CAD build for the part. Positions are in the model's coordinates, mm. Face numbers are marked on the shaded views. Give positions to 0.01 mm unless a question says otherwise; leave off trailing zeros. Loops run counter-clockwise (first coordinate to the right, second up) from the corner with the lowest first, then second, coordinate; pieces in that order, holes last. Notation, with made-up numbers: M 8.5,34 L 46.5,34 A20 ccw 46.5,40 Z; hole C 38,8 d3. An arc over 180 degrees is marked long. Answer as CSV lines item,"result".
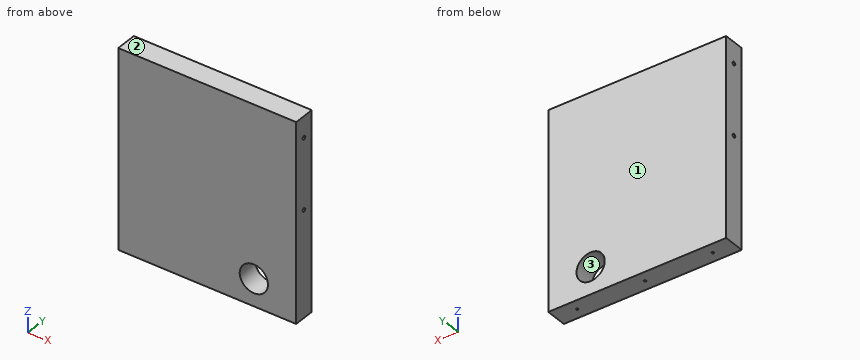
```python
from build123d import *

# Parameters (mm, degrees)
SKETCH1_W                  = 160.02
SKETCH1_H                  = 19.05
BOSS_EXTRUDE1_DEPTH        = 177.8
HOLE1_D                    = 1.98374
HOLE1_DEPTH                = 31.75
HOLE1_CSINK_D              = 10.16
HOLE1_CSINK_ANGLE          = 82
HOLE1_TIP                  = 0.595975622
HOLE3_D                    = 3.175
HOLE3_DEPTH                = 31.75
HOLE3_CSINK_D              = 10.16
HOLE3_CSINK_ANGLE          = 82
HOLE3_TIP                  = 0.953866233
HOLE4_D                    = 3.175
HOLE4_DEPTH                = 31.75
HOLE4_CSINK_D              = 10.16
HOLE4_CSINK_ANGLE          = 82
HOLE4_TIP                  = 0.953866233
F_1_1_DIAMETER_HOLE1_D     = 25.4
F_1_1_DIAMETER_HOLE1_DEPTH = 19.05


with BuildPart() as part:
    # Sketch1 → Boss-Extrude1 (new body)
    with BuildSketch(Plane.XY):
        with Locations((0, 5836.579380546)):
            Rectangle(SKETCH1_W, SKETCH1_H)
    extrude(amount=BOSS_EXTRUDE1_DEPTH)

    # Hole1
    with Locations(Plane(origin=(0, 0, -19.05), x_dir=(-1, 0, 0), z_dir=(0, 0, -1))):
        with Locations((0.162188158, 5756.275), (0, 5926.455000144), (-203.2, 5926.455000144), (-406.4, 5926.455000144), (-406.562188158, 5756.275), (-203.362188158, 5756.275), (-359.617959774, 5737.225), (-428.613879322, 5737.225), (-421.257783583, 5578.475), (-319.657783583, 5578.475), (-116.457783583, 5578.475), (-424.072610901, 5559.425), (-358.104203634, 5559.425), (-418.230271303, 5400.675), (-316.630271303, 5400.675), (-113.430271303, 5400.675), (-419.531342481, 5381.625), (-356.590447494, 5381.625), (-415.202759023, 5222.875), (-313.602759023, 5222.875), (-110.402759023, 5222.875), (-414.990074061, 5203.825), (-355.076691354, 5203.825), (355.076691354, 5203.825), (414.990074061, 5203.825), (110.402759023, 5222.875), (313.602759023, 5222.875), (415.202759023, 5222.875), (356.590447494, 5381.625), (419.531342481, 5381.625), (113.430271303, 5400.675), (316.630271303, 5400.675), (418.230271303, 5400.675), (358.104203634, 5559.425), (424.072610901, 5559.425), (116.457783583, 5578.475), (319.657783583, 5578.475), (421.257783583, 5578.475), (428.613879322, 5737.225), (359.617959774, 5737.225), (203.362188158, 5756.275), (406.562188158, 5756.275), (406.4, 5926.455000144), (203.2, 5926.455000144), (-0.162188158, 5756.275), (0, 5836.579380546), (-60.96, 5836.579380546), (60.96, 5836.579380546)):
            CounterSinkHole(HOLE1_D / 2, HOLE1_CSINK_D / 2, depth=HOLE1_DEPTH, counter_sink_angle=HOLE1_CSINK_ANGLE)
            with Locations((0, 0, -(HOLE1_DEPTH + HOLE1_TIP / 2))):  # 118° drill point
                Cone(0, HOLE1_D / 2, HOLE1_TIP, mode=Mode.SUBTRACT)

    # Hole3
    with Locations(Plane(origin=(99.06, 0, -2683.51), x_dir=(0, 0, -1), z_dir=(1, 0, 0))):
        with Locations((-2778.76, 5836.579380546), (-2842.26, 5836.579380546)):
            CounterSinkHole(HOLE3_D / 2, HOLE3_CSINK_D / 2, depth=HOLE3_DEPTH, counter_sink_angle=HOLE3_CSINK_ANGLE)
            with Locations((0, 0, -(HOLE3_DEPTH + HOLE3_TIP / 2))):  # 118° drill point
                Cone(0, HOLE3_D / 2, HOLE3_TIP, mode=Mode.SUBTRACT)

    # Hole4
    with Locations(Plane(origin=(-99.06, 0, -2683.51), x_dir=(0, 0, 1), z_dir=(-1, 0, 0))):
        with Locations((2778.76, 5836.579380546), (2842.26, 5836.579380546)):
            CounterSinkHole(HOLE4_D / 2, HOLE4_CSINK_D / 2, depth=HOLE4_DEPTH, counter_sink_angle=HOLE4_CSINK_ANGLE)
            with Locations((0, 0, -(HOLE4_DEPTH + HOLE4_TIP / 2))):  # 118° drill point
                Cone(0, HOLE4_D / 2, HOLE4_TIP, mode=Mode.SUBTRACT)

    # 1 (1) Diameter Hole1
    with Locations(Plane(origin=(0, 5827.054380546, 0), x_dir=(-1, 0, 0), z_dir=(0, -1, 0))):
        with Locations((-41.91, -24.295160427)):
            Hole(F_1_1_DIAMETER_HOLE1_D / 2, depth=F_1_1_DIAMETER_HOLE1_DEPTH)


solid = part.part
```
Q1. Pin check, flat tips, straight feed: P1, Ø5, axis at x = 16, y = 5834.5, coming from the -Z side; P2, Ø3, axis at y = 5836.58, z = 95.25, coming from the -X side; P3, Ø2.5, axis at y = 5836.58, z = 158.75, coming from the -X side. Stop position of each tip, or through.
Solution:
P1,"stops at z = 0"
P2,"stops at x = -67.26"
P3,"stops at x = -67.11"
Q2. Mould opens along Z. For the marked faces 1, 2 and 3 say: released by +Z, released by -Z, zero draft, split by the parting line, or undercut.
Solution:
face 1,"zero draft"
face 2,"released by +Z"
face 3,"undercut"
Q3. Cut at A-A (x = 41.91). Write the cut outline in (y, z).
Solution:
outline,"M 5827.05,0 L 5846.1,0 L 5846.1,11.6 L 5827.05,11.6 Z; M 5827.05,37 L 5846.1,37 L 5846.1,177.8 L 5827.05,177.8 Z"
Q4. Wall check: line 1 (Y direction, x = 73.25, z = 95.25); line 2 (Y direction, x = 70.5, z = 96); line 3 (Z direction, x = 39.5, y = 5836). Give the ranges that are in metal, low to high. Write a range as [from, to].
Solution:
line 1,"y = [5827.05, 5834.99], [5838.17, 5846.1]"
line 2,"y = [5827.05, 5835.18], [5837.98, 5846.1]"
line 3,"z = [0, 11.83], [36.76, 177.8]"
